Autodesk Inventor part; units mm, degrees
ref_plane "YZ Plane" through (0, 0, 0) normal (1, 0, 0) x (0, 1, 0)
ref_plane "XZ Plane" through (0, 0, 0) normal (0, 1, 0) x (-1, 0, 0)
ref_plane "XY Plane" through (0, 0, 0) normal (0, 0, 1) x (1, 0, 0)
sketch "Эскиз1" plane through (0, 0, 0) normal (0, 0, 1) x (1, 0, 0)
  circle A0 centre (0, 0) radius 30
  dimension "d0" = 60
extrude "Выдавливание1" add sketch "Эскиз1" against normal blind 20
sketch "Эскиз2" plane through (0, 0, -20) normal (0, 0, -1) x (-1, 0, 0)
  circle A0 centre (0, 0) radius 30
  circle A1 centre (0, 0) radius 20
  dimension "d3" = 40
extrude "Выдавливание2" add sketch "Эскиз2" along normal blind 40 contours A1
sketch "Эскиз3" plane through (0, 0, -60) normal (0, 0, -1) x (-1, 0, 0)
  circle A0 centre (0, 0) radius 20
  arc A1 (9.5394, 3) -> (9.5394, -3) centre (0, 0) ccw
  line L0 (9.5394, 3) -> (11.5, 3)
  line L1 (11.5, 3) -> (11.5, -3)
  line L2 (11.5, -3) -> (9.5394, -3)
  dimension "d6" = 20
  dimension "d8" = 11.5
  dimension "d9" = 3
  dimension "d10" = 3
extrude "Выдавливание3" cut sketch "Эскиз3" against normal through all contours L0 L1 L2 A1
fillet "Сопряжение2" radius 5 1 edges at (20, 0, -20)
properties part number "Колесо"
Model file for the job. Use its own axes, mm. A direction names the side the tool comes from. Coordinates: 2 decimals unless noted, no trailing zeros. Write each loop counter-clockwise with the first axis right and the second up, starting at its lowest first coordinate (ties: lowest second). Pieces come first, ordered by that corner, then holes. Notation, with made-up numbers: (46, 88.5) - (94, 88.5) arc R24 cw to (94, 113.5) - close; hole circle Ø8 at (76, 10). An arc over 180 degrees is marked (long way). Use a Markdown table: item, result. Add a question column.
Item 1: Band-saw the part on D-D, the plane z = -28. Write the cut outline in (x, y), and give its area (3 significant figures).
Item 2: 3-axis set-ups, long thin cutter, end or side, ignore diameter. For faces 4 (the face through (-7, 25, -20)), 5 (the face through (5, 9, -60)), 6 (the face through (-11, -3, -30)): which of +Z, -Z, +X, -X, +Y, -Y reach the whole face in a straight line?
Item 3: Band-saw the part on A-A, the plane x = 0. Write the cut outline in (y, z), and give its area (3 significant figures).
Item 4: Two-plate mould, pull along Y, no slides. Class faces 1 (the face through (-11, 3, -30)), 2 (the face through (-29.97, 1.32, -9.86)), 3 (the face through (13, 0, 0)): pulls with the +Y half, pulls with the -Y half, needs draft (parallel to the pull), parting line crosses it, or undercut.
Item 5: Drop flat-ended pins along their axis: pin 1 (12 mm diameter, centred on x = 0, y = 0, fed in from +Z); pin 2 (1.5 mm diameter, centred on y = -16, z = -12, fed in from -X); pin 3 (5 mm diameter, centred on x = 21, z = -17, fed in from -Y); pin 4 (5 mm diameter, centred on y = 11, z = -7.5, fed in from +X). Give the stop position or say it passes through.
Item 6: Band-saw the part on C-C, the plane z = -3.5. Write the cut outline in (x, y).
Item 7: Drill centre lines: line 1 along Y through (x, z) = (0, -13); line 2 along Y through (x, z) = (0.5, -27.5); line 3 along X through (y, z) = (-4.5, -50.5). Where is each one in solid material? Low to high.
Item 8: Band-saw the part on B-B, the plane y = 0. Write the cut outline in (x, z).
A:
| question | item | result |
|---|---|---|
| 1 | outline | circle Ø40 at (0, 0); hole (-11.5, -3) - (-9.54, -3) arc R10 ccw (long way) to (-9.54, 3) - (-11.5, 3) - close |
| 1 | area | 933 mm² |
| 2 | face 4 | -Z |
| 2 | face 5 | -Z, +X, -X, +Y, -Y |
| 2 | face 6 | +Z, -Z |
| 3 | outline | (-30, -20) - (-25, -20) arc R5 cw to (-20, -25) - (-20, -60) - (-10, -60) - (-10, 0) - (-30, 0) - close; (10, -60) - (20, -60) - (20, -25) arc R5 cw to (25, -20) - (30, -20) - (30, 0) - (10, 0) - close |
| 3 | area | 1,610 mm² |
| 4 | face 1 | undercut |
| 4 | face 2 | parting line crosses it |
| 4 | face 3 | needs draft |
| 5 | pin 1 | passes through |
| 5 | pin 2 | stops at x = -25.83 |
| 5 | pin 3 | stops at y = -23.62 |
| 5 | pin 4 | stops at x = 28.77 |
| 6 | outline | circle Ø60 at (0, 0); hole (-11.5, -3) - (-9.54, -3) arc R10 ccw (long way) to (-9.54, 3) - (-11.5, 3) - close |
| 7 | line 1 | y = -30 to -10, 10 to 30 |
| 7 | line 2 | y = -19.99 to -9.99, 9.99 to 19.99 |
| 7 | line 3 | x = -19.49 to -8.93, 8.93 to 19.49 |
| 8 | outline | (-30, -20) - (-25, -20) arc R5 cw to (-20, -25) - (-20, -60) - (-11.5, -60) - (-11.5, 0) - (-30, 0) - close; (10, -60) - (20, -60) - (20, -25) arc R5 cw to (25, -20) - (30, -20) - (30, 0) - (10, 0) - close |
